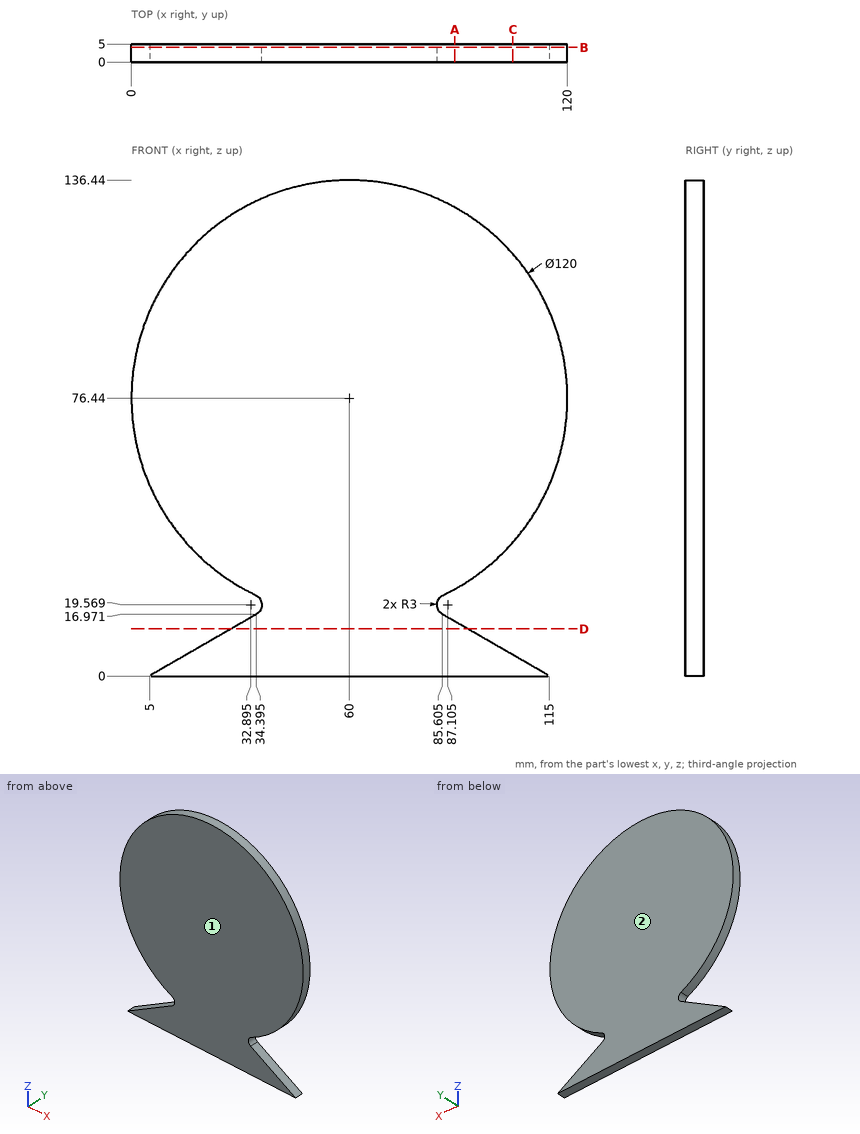
Geometry check sheet. Reference: drawing and pictorial views, mm from the part's lowest x, y, z. Coordinates: 2 decimals unless noted, no trailing zeros. Order: outer loops, then holes, each group sorted by start corner. A loop starts at its lowest first (then second) coordinate and runs counter-clockwise, first axis right, second up. Notation, with made-up numbers: (-21.5, 26) -> (8.5, 26) arc R27 ccw to (8.5, 49) -> close; hole circle Ø5 at (20.25, 32). An arc over 180 degrees is marked (long way). Put each result on its own line as item: value. Start each with the question number.
1) Go/stop test with flat-tipped pins: pin 1 (1.5 mm diameter, centred on y = 2.5, z = 120.5, fed in from +X) (1 decimal); pin 2 (3 mm diameter, centred on y = 1.5, z = 28.5, fed in from -X). Record where each tip stops, or that it passes through.
2) Cross-section at D-D (z = 13). Enter the section's corners in (x, y), plus the area to 3 significant figures.
3) Release check for a two-part mould opening along Y. For the marked faces 1 and 2 record: pulls with the +Y half, pulls with the -Y half, needs draft (parallel to the pull), parting line crosses it, or undercut.
4) Cross-section at C-C (x = 105). Enter the section's corners in (y, z), plus the area to 3 significant figures.
5) Material ranges on L1, parallel to Z at x = 102.5, y = 0.6 (1 decimal); L2, parallel to Z at x = 110.5, y = 4.75; L3, parallel to X at y = 3.9, z = 57.5, recorded low to high.
6) Cross-section at B-B (y = 4.1). Enter the section's corners in (x, z) (1 decimal).
7) Cross-section at A-A (x = 89). Enter the section's corners in (y, z).
Geometry check:
1. pin 1: stops at x = 101.5
1. pin 2: stops at x = 22.01
2. outline: (27.52, 0) -> (92.48, 0) -> (92.48, 5) -> (27.52, 5) -> close
2. area: 325 mm^2
3. face 1: pulls with the -Y half
3. face 2: pulls with the +Y half
4. outline: (0, 0) -> (5, 0) -> (5, 5.77) -> (0, 5.77) -> close; (0, 36.75) -> (5, 36.75) -> (5, 116.13) -> (0, 116.13) -> close
4. area: 426 mm^2
5. L1: z = 0 to 7.2, 34.1 to 118.8
5. L2: z = 0 to 2.6, 44.04 to 108.84
5. L3: x = 3.07 to 116.93
6. outline: (5, 0) -> (115, 0) -> (85.6, 17) arc R3 cw to (85.8, 22.3) arc R60 ccw (long way) to (34.2, 22.3) arc R3 cw to (34.4, 17) -> close
7. outline: (0, 0) -> (5, 0) -> (5, 15.01) -> (0, 15.01) -> close; (0, 23.91) -> (5, 23.91) -> (5, 128.97) -> (0, 128.97) -> close
